Verification items for the finished model (mm, model axes). Face numbers are marked on the shaded views. A direction names the side the tool comes from. Round coordinates to 2 decimals unless told otherwise and drop trailing zeros. Write each loop counter-clockwise with the first axis right and the second up, starting at its lowest first coordinate (ties: lowest second). Pieces come first, ordered by that corner, then holes.
Autodesk Inventor part; units mm, degrees
ref_plane "YZ Plane" through (0, 0, 0) normal (1, 0, 0) x (0, 1, 0)
ref_plane "XZ Plane" through (0, 0, 0) normal (0, 1, 0) x (-1, 0, 0)
ref_plane "XY Plane" through (0, 0, 0) normal (0, 0, 1) x (1, 0, 0)
sketch "Skizze1" plane through (0, 0, 0) normal (0, 1, 0) x (-1, 0, 0)
  arc A0 (20, 17) -> (15, 22) centre (15, 17) ccw
  arc A1 (-15, 22) -> (-20, 17) centre (-15, 17) ccw
  line L0 (14, -12) -> (18, -12)
  arc A2 (14, -12) -> (14, -16) centre (14, -14) ccw
  line L1 (18, -16) -> (14, -16)
  line L2 (-14, -16) -> (-18, -16)
  arc A3 (-14, -16) -> (-14, -12) centre (-14, -14) ccw
  line L3 (-18, -12) -> (-14, -12)
  line L4 (-14, 12) -> (-18, 12)
  arc A4 (-14, 12) -> (-14, 16) centre (-14, 14) ccw
  line L5 (-18, 16) -> (-14, 16)
  line L6 (14, 16) -> (18, 16)
  arc A5 (14, 16) -> (14, 12) centre (14, 14) ccw
  line L7 (18, 12) -> (14, 12)
  line L8 (14, 14) -> (-14, 14) construction
  line L9 (-14, 14) -> (-14, -14) construction
  line L10 (-14, -14) -> (14, -14) construction
  line L11 (14, -14) -> (14, 14) construction
  line L12 (14, 14) -> (-14, -14) construction
  line L13 (-14, 14) -> (14, -14) construction
  circle A6 centre (0, 0) radius 7.5
  line L14 (20, -40) -> (-20, -40) construction
  line L15 (-20, -40) -> (-20, 22) construction
  line L16 (-20, 22) -> (20, 22) construction
  line L17 (20, 22) -> (20, -40) construction
  line L18 (20, -40) -> (-20, -40)
  line L19 (15, 22) -> (-15, 22)
  line L20 (20, -40) -> (20, 17)
  line L21 (-20, 17) -> (-20, -40)
  line L22 (0, -40) -> (0, 22) construction
  arc A7 (18, 17) -> (15, 20) centre (15, 17) ccw
  arc A8 (-15, 20) -> (-18, 17) centre (-15, 17) ccw
  line L23 (-15, 20) -> (15, 20)
  circle A9 centre (14, 14) radius 0.9
  circle A10 centre (-14, 14) radius 0.9
  circle A11 centre (-14, -14) radius 0.9
  circle A12 centre (14, -14) radius 0.9
  line L24 (20, -28) -> (-20, -28)
  circle A13 centre (-15, -23) radius 5 construction
  circle A14 centre (15, -23) radius 5 construction
  line L25 (-18, -18) -> (-15, -18)
  line L26 (-10, -23) -> (-10, -26)
  line L27 (15, -18) -> (18, -18)
  line L28 (10, -23) -> (10, -26)
  arc A15 (-10, -23) -> (-15, -18) centre (-15, -23) ccw
  arc A16 (15, -18) -> (10, -23) centre (15, -23) ccw
  circle A17 centre (-15, -23) radius 2.25
  circle A18 centre (15, -23) radius 2.25
  line L29 (-18, -18) -> (-18, 17)
  line L30 (18, 17) -> (18, -18)
  line L31 (-10, -26) -> (10, -26)
  point P0 (0, 0)
  point P1 (0, 20)
  point P2 (0, -26)
  point P3 (-15, -18)
  point P4 (-12, -14)
  point P5 (-12, -19)
  point P6 (12, -14)
  point P7 (12, -19)
  dimension "d2" = 15
  dimension "d3" = 40
  dimension "d5" = 22
  dimension "d7" = 5
  dimension "d10" = 2
  dimension "d14" = 1.8
  dimension "d41" = 12
  dimension "d42" = 2
  dimension "d43" = 2
  dimension "d45" = 4.5
  dimension "d49" = 10
  dimension "d50" = 28
  dimension "d51" = 2
  dimension "d52" = 28
extrude "Extrusion1" add sketch "Skizze1" against normal blind 2 contours L20 L24 L21 A1 L19 A0 | L20 L18 L21 L24 | A2 L1 L30 L27 A16 L28 L31 L26 A15 L25 L29 L2 A3 L3 L4 A4 L5 A8 L23 A7 L6 A5 L7 L0 | L0 L30 L1 A2 | L7 A5 L6 L30 | L5 A4 L4 L29 | L3 A3 L2 L29 | A9 | A10 | A11 | A12 | A17 | A18
extrude "Extrusion2" add sketch "Skizze1" along normal blind 16 contours L20 L24 L21 A1 L19 A0
extrude "Extrusion3" add sketch "Skizze1" along normal blind 6 contours L20 L18 L21 L24
extrude "Extrusion4" add sketch "Skizze1" along normal blind 6.5 contours L0 L30 L1 A2 | L7 A5 L6 L30 | L5 A4 L4 L29 | L3 A3 L2 L29
sketch "Skizze2" plane through (0, -2, 0) normal (0, -1, 0) x (1, 0, 0)
  arc A0 (-15, 22) -> (-20, 17) centre (-15, 17) ccw
  line L0 (-20, 17) -> (-20, -40)
  line L1 (-20, -40) -> (20, -40)
  line L2 (20, -40) -> (20, 17)
  arc A1 (20, 17) -> (15, 22) centre (15, 17) ccw
  line L3 (15, 22) -> (-15, 22)
  circle A2 centre (0, 0) radius 7.5
  line L4 (15, 22) -> (-15, 22)
  line L5 (0, 22) -> (0, -40) construction
  point P0 (10, -34)
  point P1 (-10, -34)
  dimension "d25" = 20
  dimension "d26" = 6
hole "Bohrung1" at (10, -2, -34) at (-10, -2, -34) direction (0, 1, 0) diameter 3.2 end through all counterbore diameter 6.5 counterbore depth 3.4
sketch "Skizze3" plane through (20, -2, -40) normal (0, 0, -1) x (-1, 0, 0)
  line L0 (0, 8) -> (40, 8)
  line L1 (40, 8) -> (40, 18)
  line L2 (0, 18) -> (40, 18)
  line L3 (0, 8) -> (0, 18)
  line L4 (0, 0) -> (0, 8)
  line L5 (40, 0) -> (0, 0)
  line L6 (40, 0) -> (40, 8)
  line L7 (0, 8) -> (40, 8)
  line L8 (0, 8) -> (40, 8)
  ellipse E0 centre (20, 8) end of major axis (25, 8) minor radius 3
  line L9 (0, 8) -> (40, 8)
  line L10 (15, 8) -> (15, 18)
  line L11 (5, 18) -> (35, 18)
  line L12 (15, 18) -> (25, 18)
  line L13 (25, 8) -> (25, 18)
  point P0 (20, 2)
  dimension "d37" = 3
  dimension "d38" = 5
extrude "Extrusion5" cut sketch "Skizze3" against normal up to surface (14 mm away) contours E0 L0 | L10 L2 L13 E0 | L0 E0
extrude "Extrusion6" add sketch "Skizze1" along normal blind 10 contours A17 | A18
chamfer "Fase1" distance 1 angle 45 5 edges at (20, -2, -11.5) (18.5355, -2, 20.5355) (0, -2, 22) (-18.5355, -2, 20.5355) (-20, -2, -11.5)
equation "\"d42\" = d51"
equation "\"d43\" = d51"
properties part number "LED-Ring_Camera-Housing"
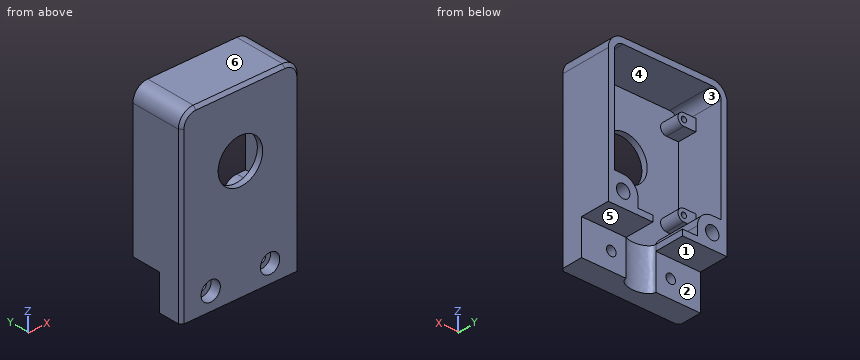
Q1. Tool access check on the marked faces 4, 5 and 6. Record the directions out of +Z, -Z, +X, -X, +Y, -Y that give a thin tool (end or side, any length) a straight path to the whole face; none if there is none.
Recorded:
face 4: +Y
face 5: -Z, +X, -X, +Y
face 6: +Z, +X, -X, +Y, -Y
Q2. Release check for a two-part mould opening along Z. For the marked faces 1, 2 and 3 record: released by +Z, released by -Z, zero draft, split by the parting line, or undercut.
Recorded:
face 1: released by -Z
face 2: zero draft
face 3: undercut
Q3. Sectioned sample at A-A (z = 6.5). Enter the section's corners in (x, y), plus the area to 3 significant figures.
Recorded:
outline: (-20, -1) - (-19, -2) - (-3.74, -2) - (-3.74, 0) - (-18, 0) - (-18, 16) - (-20, 16) - close; (3.74, -2) - (19, -2) - (20, -1) - (20, 16) - (18, 16) - (18, 0) - (3.74, 0) - close
area: 128 mm2
Q4. Sectioned sample at B-B (z = -34). Give the number of separate pieces and of enclosed holes in the cut face, plus the area to 3 significant figures.
Recorded:
separate pieces: 3
enclosed holes: 0
area: 222 mm2
Q5. Sectioned sample at C-C (z = -14). Enter the section's corners in (x, y), plus the area to 3 significant figures.
Recorded:
outline: (-20, -1) - (-19, -2) - (19, -2) - (20, -1) - (20, 16) - (18, 16) - (18, 6.5) - (14.9, 6.5) - (14.9, 0) - (13.1, 0) - (13.1, 6.5) - (12, 6.5) - (12, 0) - (-12, 0) - (-12, 6.5) - (-13.1, 6.5) - (-13.1, 0) - (-14.9, 0) - (-14.9, 6.5) - (-18, 6.5) - (-18, 16) - (-20, 16) - close
area: 198 mm2
Q6. Material ranges on line 1 along Z through (x, y) = (11, 6.25); line 2 along X through (y, z) = (9, -1); line 3 along X through (y, z) = (4.5, -14.5), recorded low to high.
Recorded:
line 1: z = -28 to -20, 20 to 22
line 2: x = -20 to -18, 18 to 20
line 3: x = -20 to -14.75, -13.25 to -12.06, 12.06 to 13.25, 14.75 to 20
Q7. Depth check by flat-ended pin: P1, Ø3.5, axis at x = -9.5, z = -32.5, coming from the +Y side; P2, Ø4.5, axis at x = -15.5, z = 13, coming from the +Y side; P3, Ø4, axis at x = -8, y = 12, coming from the -Z side; P4, Ø1, axis at x = 2.5, z = -5.5, coming from the -Y side. Enter the tip coordinate at first touch or a pass-through.
Recorded:
P1: stops at y = 6
P2: stops at y = 6.5
P3: stops at z = -28
P4: passes through
